Geometry check sheet. Reference: the model listing, model coordinates, mm. Face numbers are marked on the shaded views. A direction names the side the tool comes from. Round coordinates to 2 decimals unless told otherwise and drop trailing zeros. Write each loop counter-clockwise with the first axis right and the second up, starting at its lowest first coordinate (ties: lowest second). Pieces come first, ordered by that corner, then holes. Notation, with made-up numbers: (76, 71) - (95, 71) arc R17 cw to (95, 95) - close; hole circle Ø5 at (61, 68). An arc over 180 degrees is marked (long way). One line per question, with ' | ' between items. Start each with the question number.
from build123d import *

# Parameters (mm, degrees)
F1_DEPTH = 482.6
F3_DEPTH = 76.201
F4_R     = 10.3124
F5_DEPTH = 76.201
F6_R     = 5.08


with BuildPart() as f1:
    # F0 (on Top) → F1 (new body, symmetric)
    with BuildSketch(Plane.XY):
        Polygon((0, 76.2), (0, 0), (6.35, 0), (6.35, 69.85), (76.2, 69.85), (76.2, 76.2), align=None)
    extrude(amount=F1_DEPTH, both=True)

    # F2 (on Front) → F3 (cut, through all)
    with BuildSketch(Plane.XZ):
        Polygon((84.518964, -404.431036), (6.35, -482.6), (84.518964, -482.6), align=None)
    extrude(amount=-F3_DEPTH, mode=Mode.SUBTRACT)

    # F4 (on Right) → F5 (cut, through all)
    with BuildSketch(Plane.YZ):
        with Locations((38.1, -438.15)):
            Circle(F4_R)
        with Locations((38.1, 431.8)):
            Circle(F4_R)
    extrude(amount=F5_DEPTH, mode=Mode.SUBTRACT)

    # F6
    f6_edges = [f1.edges().sort_by_distance(p)[0] for p in [
        (6.35, 69.85, 0),
        (76.2, 69.85, 34.925),
        (6.35, 0, 0),
    ]]
    fillet(f6_edges, radius=F6_R)


solid = f1.part
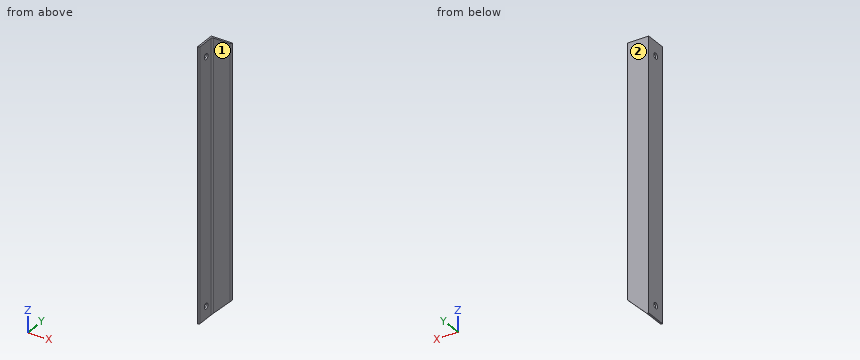
Q1. Section check C-C, the plane z = -263. Record the cut outline in (x, y), then the cut area to 3 significant figures.
Q2. Go/stop test with flat-tipped pins: P1, Ø12, axis at y = 32.5, z = 6.5, coming from the +X side; P2, Ø6, axis at y = 10.5, z = 82.5, coming from the +X side; P3, Ø18.5, axis at y = 38.1, z = -438.15, coming from the -X side; P4, Ø1, axis at x = 18.5, z = 129, coming from the -Y side. Record where each tip stops, or that it passes through.
Q3. Thickness scan on line 1 (Z direction, x = 2.5, y = 38.1); line 2 (X direction, y = 27, z = 412); line 3 (Y direction, x = 53, z = -228). Record the ranges inside material, lowest first.
Q4. Section check D-D, the plane z = -438.15. Record the cut outline in (x, y).
Q5. Set-up check for the marked faces 1 and 2: record each of +Z, -Z, +X, -X, +Y, -Y from which the full face is reachable in a straight line by a thin tool's end or side.
Q6. Section check A-A, the plane z = 431.8. Record the cut outline in (x, y), then the cut area to 3 significant figures.
Q7. Section check B-B, the plane y = 38.1. Record the cut outline in (x, z).
Result sheet:
1) outline: (0, 0) - (1.27, 0) arc R5.08 ccw to (6.35, 5.08) - (6.35, 64.77) arc R5.08 cw to (11.43, 69.85) - (71.12, 69.85) arc R5.08 ccw to (76.2, 74.93) - (76.2, 76.2) - (0, 76.2) - close | area: 922 mm²
2) P1: x = 6.35 | P2: x = 6.35 | P3: through | P4: y = 69.85
3) line 1: -482.6 to -448.46, -427.84 to 421.49, 442.11 to 482.6 | line 2: 0 to 6.35 | line 3: 69.85 to 76.2
4) outline: (0, 0) - (1.27, 0) arc R5.08 ccw to (6.35, 5.08) - (6.35, 27.79) - (0, 27.79) - close; (0, 48.41) - (6.35, 48.41) - (6.35, 64.77) arc R5.08 cw to (11.43, 69.85) - (50.8, 69.85) - (50.8, 76.2) - (0, 76.2) - close
5) face 1: +Z, -Z, +X, -Y | face 2: +Z, -Z, +X, -X, +Y
6) outline: (0, 0) - (1.27, 0) arc R5.08 ccw to (6.35, 5.08) - (6.35, 27.79) - (0, 27.79) - close; (0, 48.41) - (6.35, 48.41) - (6.35, 64.77) arc R5.08 cw to (11.43, 69.85) - (71.12, 69.85) arc R5.08 ccw to (76.2, 74.93) - (76.2, 76.2) - (0, 76.2) - close | area: 791 mm²
7) outline: (0, -482.6) - (6.35, -482.6) - (6.35, -448.46) - (0, -448.46) - close; (0, -427.84) - (6.35, -427.84) - (6.35, 421.49) - (0, 421.49) - close; (0, 442.11) - (6.35, 442.11) - (6.35, 482.6) - (0, 482.6) - close
